Verification items for the finished model (mm, model axes). Coordinates: 2 decimals unless noted, no trailing zeros. Loops run counter-clockwise (first coordinate to the right, second up) from the corner with the lowest first, then second, coordinate; pieces in that order, holes last. Notation, with made-up numbers: (-14.75, -36.75) - (1.25, -36.75) arc R9 ccw to (1.25, -22.75) - close; hole circle Ø8 at (54.5, -24). An arc over 180 degrees is marked (long way). One line per item, written item: value. Start each with the question number.
(1) Gauge pin test, flat ends, axial feed: P1, Ø3.5, axis at x = -8, z = -8, coming from the -Y side; P2, Ø2, axis at y = 4.5, z = -28, coming from the +X side; P3, Ø2, axis at x = 14, y = 2.5, coming from the +Z side; P4, Ø1, axis at y = 2, z = 11, coming from the +X side. Record the tip position at first contact, or that the pin passes through.
(2) Section check A-A (x = 0). Record the boundary of the cut face in (y, z) (3 decimals), plus the area to 3 significant figures.
(3) Section check C-C (x = 36). Record the boundary of the cut face in (y, z), plus the area to 3 significant figures.
(4) Section check D-D (z = 48). Record the boundary of the cut face in (x, y).
(5) Draft check along Z on faces 1 (the face through (-5.77, 3.22, 7.71)), 2 (the face through (-15, 6.35, -1)), 3 (the face through (21.935, 3.131, 69.653)). Enter one of: +Z half, -Z half, draft (parallel to the pull), parting line (faces both ways), or undercut.
(6) Section check B-B (y = 3.75). Count the separate pieces of the cut face and the enclosed holes in it, plus the area to 3 significant figures.
(7) Thickness scan on probe 1 along X at (y, z) = (4.75, 10.5); probe 2 along X at (y, z) = (2.25, 17.78); probe 3 along Z at (x, y) = (6, 4.25). Record the ranges inside material, lowest first. Write a range as [from, to].
```python
from build123d import *

# Parameters (mm, degrees)
SKETCH1_R           = 73.025
BOSS_EXTRUDE1_DEPTH = 6.35
SKETCH2_R           = 7.5
CUT_EXTRUDE1_DEPTH  = 104.467984179
SKETCH3_R           = 2.25
CUT_EXTRUDE2_DEPTH  = 104.467984179
SKETCH4_R           = 12.7
CUT_EXTRUDE3_DEPTH  = 104.467984179
SKETCH5_R           = 1.25
CUT_EXTRUDE4_DEPTH  = 104.467984179
SKETCH6_R           = 2.5
SKETCH6_R_2         = 2.2225
CUT_EXTRUDE5_DEPTH  = 104.467984179


with BuildPart() as part:
    # Sketch1 → Boss-Extrude1 (new body)
    with BuildSketch(Plane(origin=(0, 0, 0), x_dir=(1, 0, 0), z_dir=(0, 1, 0))):
        with Locations(Location((0, 0, 0), (0, 0, 270))):
            Circle(SKETCH1_R)
    extrude(amount=BOSS_EXTRUDE1_DEPTH)

    # Sketch2 → Cut-Extrude1 (cut, through all)
    with BuildSketch(Plane(origin=(0, 6.35, 0), x_dir=(1, 0, 0), z_dir=(0, 1, 0))):
        with Locations(Location((0, 0, 0), (0, 0, 270))):
            Circle(SKETCH2_R)
    extrude(amount=-CUT_EXTRUDE1_DEPTH, mode=Mode.SUBTRACT)

    # Sketch3 → Cut-Extrude2 (cut, through all)
    with BuildSketch(Plane(origin=(0, 6.35, 0), x_dir=(1, 0, 0), z_dir=(0, 1, 0))):
        with Locations(Location((-8, 8, 0), (0, 0, 270))):
            Circle(SKETCH3_R)
        with Locations(Location((8, 8, 0), (0, 0, 270))):
            Circle(SKETCH3_R)
        with Locations(Location((8, -8, 0), (0, 0, 270))):
            Circle(SKETCH3_R)
        with Locations(Location((-8, -8, 0), (0, 0, 270))):
            Circle(SKETCH3_R)
    extrude(amount=-CUT_EXTRUDE2_DEPTH, mode=Mode.SUBTRACT)

    # Sketch4 → Cut-Extrude3 (cut, through all)
    with BuildSketch(Plane.XZ):
        with Locations(Location((43.43418184, 0, 0), (0, 0, 270))):
            Circle(SKETCH4_R)
    extrude(amount=-CUT_EXTRUDE3_DEPTH, mode=Mode.SUBTRACT)

    # Sketch5 → Cut-Extrude4 (cut, through all)
    with BuildSketch(Plane.XZ):
        with BuildLine():
            ThreePointArc((-25.717186912, 42.1), (-27.817186912, 40), (-25.717186912, 37.9))
            ThreePointArc((-25.717186912, 37.9), (-24.232262671, 38.51507576), (-23.617186912, 40))
            ThreePointArc((-23.617186912, 40), (-24.232262671, 41.48492424), (-25.717186912, 42.1))
        make_face()
        with Locations(Location((-57.46, 17.78, 0), (0, 0, 270))):
            Circle(SKETCH5_R)
        with BuildLine():
            ThreePointArc((-38.095362557, 9.539806393), (-39.470362557, 10.914806393), (-40.845362557, 9.539806393))
            ThreePointArc((-40.845362557, 9.539806393), (-39.470362557, 8.164806393), (-38.095362557, 9.539806393))
        make_face()
        with Locations(Location((-35.87, 2.54, 0), (0, 0, 270))):
            Circle(SKETCH5_R)
        with Locations(Location((-57.46, 2.54, 0), (0, 0, 270))):
            Circle(SKETCH5_R)
        with BuildLine():
            ThreePointArc((-38.095362557, 58.539806393), (-39.470362557, 59.914806393), (-40.845362557, 58.539806393))
            ThreePointArc((-40.845362557, 58.539806393), (-39.470362557, 57.164806393), (-38.095362557, 58.539806393))
        make_face()
        with BuildLine():
            ThreePointArc((17.154637443, 58.539806393), (18.529637443, 57.164806393), (19.904637443, 58.539806393))
            ThreePointArc((19.904637443, 58.539806393), (18.529637443, 59.914806393), (17.154637443, 58.539806393))
        make_face()
        with BuildLine():
            ThreePointArc((25.717186912, 41.8), (23.917186912, 40), (25.717186912, 38.2))
            ThreePointArc((25.717186912, 38.2), (26.989979118, 38.727207794), (27.517186912, 40))
            ThreePointArc((27.517186912, 40), (26.989979118, 41.272792206), (25.717186912, 41.8))
        make_face()
        with BuildLine():
            ThreePointArc((19.904637443, 9.539806393), (18.529637443, 10.914806393), (17.154637443, 9.539806393))
            ThreePointArc((17.154637443, 9.539806393), (18.529637443, 8.164806393), (19.904637443, 9.539806393))
        make_face()
        with Locations(Location((-35.87, 17.78, 0), (0, 0, 270))):
            Circle(SKETCH5_R)
    extrude(amount=-CUT_EXTRUDE4_DEPTH, mode=Mode.SUBTRACT)

    # Sketch6 → Cut-Extrude5 (cut, through all)
    # profile 1 of 6: a face of its own
    with BuildSketch(Plane(origin=(0, 6.35, 0), x_dir=(1, 0, 0), z_dir=(0, 1, 0))):
        with Locations(Location((-34.460546587, 51.030675215, 0), (0, 0, 270))):
            Circle(SKETCH6_R)
        with Locations((-34.460546587, 51.030675215)):
            Circle(SKETCH6_R_2, mode=Mode.SUBTRACT)
    # profile 2 of 6: a face of its own
    with BuildSketch(Plane(origin=(0, 6.35, 0), x_dir=(1, 0, 0), z_dir=(0, 1, 0))):
        with Locations((-34.460546587, 51.030675215)):
            Circle(SKETCH6_R_2)
    # profile 3 of 6: a face of its own
    with BuildSketch(Plane(origin=(0, 6.35, 0), x_dir=(1, 0, 0), z_dir=(0, 1, 0))):
        with Locations(Location((29.018504419, 49.399698988, 0), (0, 0, 270))):
            Circle(SKETCH6_R)
        with Locations((29.018504419, 49.399698988)):
            Circle(SKETCH6_R_2, mode=Mode.SUBTRACT)
    # profile 4 of 6: a face of its own
    with BuildSketch(Plane(origin=(0, 6.35, 0), x_dir=(1, 0, 0), z_dir=(0, 1, 0))):
        with Locations((29.018504419, 49.399698988)):
            Circle(SKETCH6_R_2)
    # profile 5 of 6: a face of its own
    with BuildSketch(Plane(origin=(0, 6.35, 0), x_dir=(1, 0, 0), z_dir=(0, 1, 0))):
        with Locations(Location((-23.004278318, 2.460401205, 0), (0, 0, 270))):
            Circle(SKETCH6_R)
        with Locations((-23.004278318, 2.460401205)):
            Circle(SKETCH6_R_2, mode=Mode.SUBTRACT)
    # profile 6 of 6: a face of its own
    with BuildSketch(Plane(origin=(0, 6.35, 0), x_dir=(1, 0, 0), z_dir=(0, 1, 0))):
        with Locations((-23.004278318, 2.460401205)):
            Circle(SKETCH6_R_2)
    extrude(amount=-CUT_EXTRUDE5_DEPTH, mode=Mode.SUBTRACT)


solid = part.part
```
Responses:
1. P1: passes through
1. P2: stops at x = 67.85
1. P3: stops at z = 71.86
1. P4: stops at x = 72.27
2. outline: (0, -73.025) - (6.35, -73.025) - (6.35, -7.5) - (0, -7.5) - close; (0, 7.5) - (6.35, 7.5) - (6.35, 73.025) - (0, 73.025) - close
2. area: 832 mm²
3. outline: (0, -63.53) - (6.35, -63.53) - (6.35, -10.3) - (0, -10.3) - close; (0, 10.3) - (6.35, 10.3) - (6.35, 63.53) - (0, 63.53) - close
3. area: 676 mm²
4. outline: (-55.03, 0) - (55.03, 0) - (55.03, 6.35) - (-55.03, 6.35) - close
5. face 1: undercut
5. face 2: draft
5. face 3: parting line
6. separate pieces: 1
6. enclosed holes: 19
6. area: 15,900 mm²
7. probe 1: x = [-72.27, -40.45], [-38.49, 17.55], [19.51, 36.29], [50.58, 72.27]
7. probe 2: x = [-70.83, -58.71], [-56.21, -37.12], [-34.62, 70.83]
7. probe 3: z = [-72.78, -9.03], [-6.97, -4.5], [4.5, 6.97], [9.03, 72.78]
